Geometry check sheet. Reference: the model listing, model coordinates, mm. Face numbers are marked on the shaded views. A direction names the side the tool comes from. Round coordinates to 2 decimals unless told otherwise and drop trailing zeros. Order: outer loops, then holes, each group sorted by start corner. A loop starts at its lowest first (then second) coordinate and runs counter-clockwise, first axis right, second up. Notation, with made-up numbers: (3.5, -7.5) -> (58.5, -7.5) arc R27 cw to (58.5, 20.5) -> close; hole circle Ø9 at (13, -15.5). An arc over 180 degrees is marked (long way). Use a Markdown table: item, result. Add a question column.
Item 1: Sectioned sample at B-B, the plane z = -24. Record the cut outline in (x, y).
Item 2: Gauge pin test, flat ends, axial feed: pin 1 Ø3 at (y, z) = (-2.5, 56) entering from +X; pin 2 Ø3.5 at (y, z) = (-4, -30) entering from +X; pin 3 Ø5 at (x, z) = (4, 16) entering from +Y. Record the tip position at first contact, or that the pin passes through.
Item 3: Set-up check for the marked faces 1 and 2: record each of +Z, -Z, +X, -X, +Y, -Y from which the full face is reachable in a straight line by a thin tool's end or side.
Item 4: Material ranges on probe 1 along X at (y, z) = (2.75, -14.5); probe 2 along Y at (x, z) = (-3, 37.5); probe 3 along Y at (x, z) = (0, -21), recorded low to high. Write a range as [from, to].
Item 5: Sectioned sample at A-A, the plane z = 52.5. Record the cut outline in (x, y), and give its area (3 significant figures).
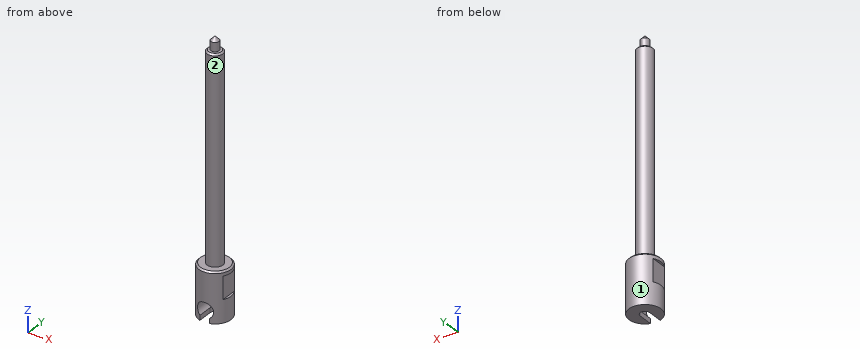
from build123d import *

# Parameters (mm, degrees)
F0_R      = 5
F1_DEPTH  = 127
F2_R      = 2.5
F3_DEPTH  = 8
F4_SIZE   = 2.5
F5_SIZE   = 1
F6_R      = 10
F6_R_2    = 5
F7_DEPTH  = 31
F9_R      = 5
F10_DEPTH = 15
F12_DEPTH = 8
F13_SIZE  = 1
F15_W     = 11.5
F15_H     = 14
F16_DEPTH = 1.5


# Not quite as in the source:
# - a pattern or mirror of a feature is missing from the dataset's text; its kind, count and spacing are read off the source's solid


with BuildPart() as f1:
    # F0 (on Top) → F1 (new body)
    with BuildSketch(Plane.XY):
        Circle(F0_R)
    extrude(amount=F1_DEPTH)

    # F2 (on face) → F3 (join)
    with BuildSketch(Plane.XY.offset(127)):
        Circle(F2_R)
    extrude(amount=F3_DEPTH)

    # F4
    f4_edges = [f1.edges().sort_by_distance(p)[0] for p in [
        (-2.5, 0, 135),
    ]]
    chamfer(f4_edges, length=F4_SIZE)

    # F5
    f5_edges = [f1.edges().sort_by_distance(p)[0] for p in [
        (-5, 0, 127),
    ]]
    chamfer(f5_edges, length=F5_SIZE)

    # F6 (on face) → F7 (join)
    with BuildSketch(Plane(origin=(0, 0, 0), x_dir=(1, 0, 0), z_dir=(0, 0, -1))):
        Circle(F6_R)
        Circle(F6_R_2, mode=Mode.SUBTRACT)
        Circle(F6_R_2)
    extrude(amount=F7_DEPTH)

    # F9 (on offset) → F10 (cut)
    with BuildSketch(Plane.XZ.offset(10)):
        with Locations((0, -24)):
            Circle(F9_R)
    extrude(amount=-F10_DEPTH, mode=Mode.SUBTRACT)

    # F11 (on face) → F12 (cut)
    with BuildSketch(Plane(origin=(0, 0, -31), x_dir=(1, 0, 0), z_dir=(0, 0, -1))):
        with BuildLine():
            Line((-3, 9.5393920142), (-3, 0))
            ThreePointArc((-3, 0), (0, -3), (3, 0))
            Line((3, 0), (3, 9.5393920142))
            ThreePointArc((3, 9.5393920142), (0, 10), (-3, 9.5393920142))
        make_face()
    extrude(amount=-F12_DEPTH, mode=Mode.SUBTRACT)

    # F13
    f13_edges = [f1.edges().sort_by_distance(p)[0] for p in [
        (-10, 0, 0),
    ]]
    chamfer(f13_edges, length=F13_SIZE)

    # F15 (on offset) → F16 (cut)
    with BuildSketch(Plane.YZ.offset(10)):
        with Locations((0, -10)):
            Rectangle(F15_W, F15_H)
    f16 = extrude(amount=-F16_DEPTH, mode=Mode.SUBTRACT)

    # F16_copies: F16 across plane
    add(f16.mirror(Plane(origin=(0, 0, 0), x_dir=(0, 0, -1), z_dir=(-1, 0, 0))), mode=Mode.SUBTRACT)


solid = f1.part
Found:
| question | item | result |
|---|---|---|
| 1 | outline | (-5, -8.66) -> (-5, 5) -> (5, 5) -> (5, -8.66) arc R10 ccw (long way) to start |
| 2 | pin 1 | stops at x = 4.9 |
| 2 | pin 2 | stops at x = 9.74 |
| 2 | pin 3 | stops at y = 4.77 |
| 3 | face 1 | +Z, -Z |
| 3 | face 2 | +Z |
| 4 | probe 1 | x = [-8.5, 8.5] |
| 4 | probe 2 | y = [-4, 4] |
| 4 | probe 3 | y = [5, 10] |
| 5 | outline | circle Ø10 at (0, 0) |
| 5 | area | 78.5 mm2 |
